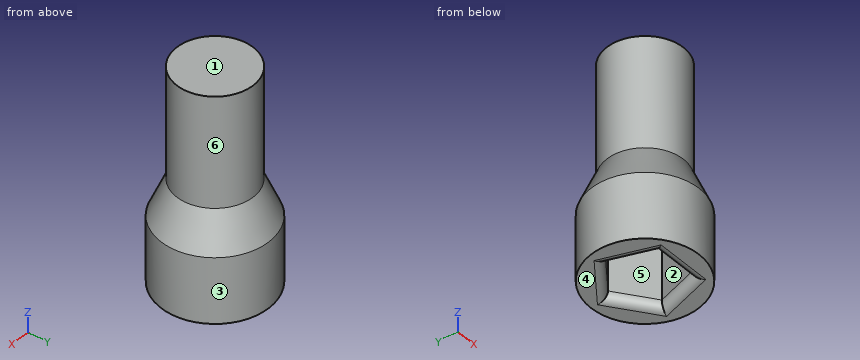
from build123d import *

# Parameters (mm, degrees)
F0_R      = 6.3393732753
F1_DEPTH  = 7.2
F2_R      = 6.3393732753
F3_DEPTH  = 0.5
F3_FACE_R = 6.3393732753
F5_R      = 4.5
F7_DEPTH  = 13
F8_R      = 1


with BuildPart() as f1:
    # F0 (on Top) → F1 (new body)
    with BuildSketch(Plane.XY):
        Circle(F0_R)
        Polygon((-2.5506196154, -3.5106267247), (-4.1269892301, 1.340940087), (0, 4.3393732753), (4.1269892301, 1.340940087), (2.5506196154, -3.5106267247), align=None, mode=Mode.SUBTRACT)
    extrude(amount=F1_DEPTH)

    # F2 (on face) → F3 (join)
    with BuildSketch(Plane.XY.offset(7.2)):
        Circle(F2_R)
        Polygon((2.5506196154, -3.5106267247), (-2.5506196154, -3.5106267247), (-4.1269892301, 1.340940087), (0, 4.3393732753), (4.1269892301, 1.340940087), align=None, mode=Mode.SUBTRACT)
        Polygon((-4.1269892301, 1.340940087), (-2.5506196154, -3.5106267247), (2.5506196154, -3.5106267247), (4.1269892301, 1.340940087), (0, 4.3393732753), align=None)
    extrude(amount=F3_DEPTH)

    # F3_face (on face) → F6 section 0
    with BuildSketch(Plane.XY.offset(7.7)):
        Circle(F3_FACE_R)
    # F5 (on offset) → F6 section 1
    with BuildSketch(Plane.XY.offset(12)):
        Circle(F5_R)
    loft()

    # F7 (add): a face of the model
    f7_faces = [f1.faces().sort_by_distance(p)[0] for p in [
        (0, 0, 12),
    ]]
    extrude(f7_faces, amount=F7_DEPTH)

    # F8
    f8_edges = [f1.edges().sort_by_distance(p)[0] for p in [
        (-3.338804, -1.084843, 0),
        (0, -3.510627, 0),
        (3.338804, -1.084843, 0),
        (2.063495, 2.840157, 0),
        (-2.063495, 2.840157, 0),
    ]]
    fillet(f8_edges, radius=F8_R)


solid = f1.part
CAD build for the part. Positions are in the model's coordinates, mm. Face numbers are marked on the shaded views. A direction names the side the tool comes from. Give positions to 0.01 mm unless a question says otherwise; leave off trailing zeros. Order: outer loops, then holes, each group sorted by start corner. A loop starts at its lowest first (then second) coordinate and runs counter-clockwise, first axis right, second up. Notation, with made-up numbers: (-31.5, 22) - (20.5, 22) arc R36 cw to (20.5, 58) - close; hole circle Ø8 at (26.25, 75.5). An arc over 180 degrees is marked (long way). Write each question's results on one line, items separated by ' | '.
1. Probe L1, parallel to Z at x = 2.25, y = 0; L2, parallel to Y at x = -2, z = 4; L3, parallel to X at y = 3, z = 4. List the from-to ranges inside material, lowest first. Write a range as from..to.
Calculated:
L1: z = 7.2..25 | L2: y = -6.02..-3.51, 2.89..6.02 | L3: x = -5.58..-1.84, 1.84..5.58
2. Pin check, flat tips, straight feed: pin 1 (1 mm diameter, centred on x = -1.5, z = 13.5, fed in from +Y); pin 2 (1 mm diameter, centred on x = 2, y = -2, fed in from -Z); pin 3 (1 mm diameter, centred on x = -1.5, z = 20.5, fed in from -Y). Stop position of each tip, or through.
Calculated:
pin 1: stops at y = 4.39 | pin 2: stops at z = 7.2 | pin 3: stops at y = -4.39
3. 3-axis set-ups, long thin cutter, end or side, ignore diameter. For the marked faces 4, 5 and 6: which of +Z, -Z, +X, -X, +Y, -Y reach the whole face in a straight line?
Calculated:
face 4: -Z, +X, -X, +Y, -Y | face 5: -Z | face 6: +Z
4. Saw through at A-A on z = 14.5. List the corners of the cut face in (x, y).
Calculated:
outline: circle Ø9 at (0, 0)
5. Pull direction Y, two halves, no side cores. Call the marked faces 1, 2 and 3: released by +Y, released by -Y, zero draft, split by the parting line, or undercut.
Calculated:
face 1: zero draft | face 2: undercut | face 3: split by the parting line
6. Saw through at B-B on z = 9.5. List the corners of the cut face in (x, y), and give its area (3 significant figures).
Calculated:
outline: circle Ø11.14 at (0, 0) | area: 97.4 mm2
